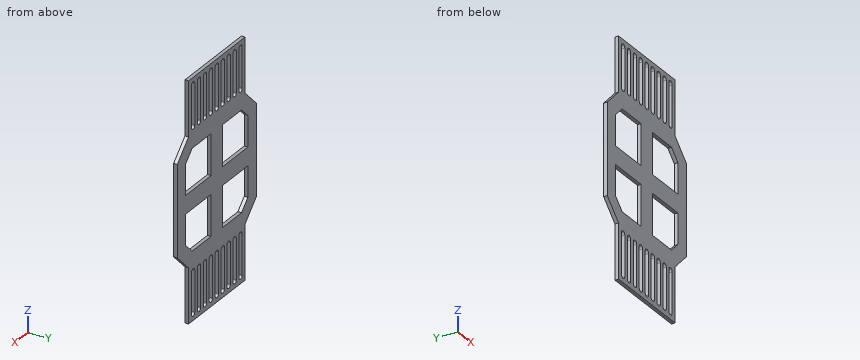
```python
from build123d import *

# Parameters (mm, degrees)
BOSS_EXTRUDE1_DEPTH = 2
CUT_EXTRUDE1_DEPTH  = 2
CIRPATTERN1_COUNT   = 4


with BuildPart() as part:
    # Sketch2 → Boss-Extrude1 (new body)
    with BuildSketch(Plane(origin=(0, 0, 0), x_dir=(1, 0, 0), z_dir=(0, 1, 0))):
        Polygon((-35, 35), (-25, 35), (-25, 65), (25, 65), (25, 35), (35, 35), (35, -35), (25, -35), (25, -65), (-25, -65), (-25, -35), (-35, -35), align=None)
        with BuildLine():
            Line((-1.5, 38.847241674), (-1.5, 61.152758326))
            ThreePointArc((-1.5, 61.152758326), (0, 62.652758326), (1.5, 61.152758326))
            Line((1.5, 61.152758326), (1.5, 38.847241674))
            ThreePointArc((1.5, 38.847241674), (0, 37.347241674), (-1.5, 38.847241674))
        make_face(mode=Mode.SUBTRACT)
        with BuildLine():
            Line((3.75, 38.847241674), (3.75, 61.152758326))
            ThreePointArc((3.75, 61.152758326), (5.25, 62.652758326), (6.75, 61.152758326))
            Line((6.75, 61.152758326), (6.75, 38.847241674))
            ThreePointArc((6.75, 38.847241674), (5.25, 37.347241674), (3.75, 38.847241674))
        make_face(mode=Mode.SUBTRACT)
        with BuildLine():
            Line((9, 38.847241674), (9, 61.152758326))
            ThreePointArc((9, 61.152758326), (10.5, 62.652758326), (12, 61.152758326))
            Line((12, 61.152758326), (12, 38.847241674))
            ThreePointArc((12, 38.847241674), (10.5, 37.347241674), (9, 38.847241674))
        make_face(mode=Mode.SUBTRACT)
        with BuildLine():
            Line((14.25, 38.847241674), (14.25, 61.152758326))
            ThreePointArc((14.25, 61.152758326), (15.75, 62.652758326), (17.25, 61.152758326))
            Line((17.25, 61.152758326), (17.25, 38.847241674))
            ThreePointArc((17.25, 38.847241674), (15.75, 37.347241674), (14.25, 38.847241674))
        make_face(mode=Mode.SUBTRACT)
        with BuildLine():
            Line((19.5, 38.847241674), (19.5, 61.152758326))
            ThreePointArc((19.5, 61.152758326), (21, 62.652758326), (22.5, 61.152758326))
            Line((22.5, 61.152758326), (22.5, 38.847241674))
            ThreePointArc((22.5, 38.847241674), (21, 37.347241674), (19.5, 38.847241674))
        make_face(mode=Mode.SUBTRACT)
        with BuildLine():
            Line((-6.75, 38.847241674), (-6.75, 61.152758326))
            ThreePointArc((-6.75, 61.152758326), (-5.25, 62.652758326), (-3.75, 61.152758326))
            Line((-3.75, 61.152758326), (-3.75, 38.847241674))
            ThreePointArc((-3.75, 38.847241674), (-5.25, 37.347241674), (-6.75, 38.847241674))
        make_face(mode=Mode.SUBTRACT)
        with BuildLine():
            Line((-12, 38.847241674), (-12, 61.152758326))
            ThreePointArc((-12, 61.152758326), (-10.5, 62.652758326), (-9, 61.152758326))
            Line((-9, 61.152758326), (-9, 38.847241674))
            ThreePointArc((-9, 38.847241674), (-10.5, 37.347241674), (-12, 38.847241674))
        make_face(mode=Mode.SUBTRACT)
        with BuildLine():
            Line((-17.25, 38.847241674), (-17.25, 61.152758326))
            ThreePointArc((-17.25, 61.152758326), (-15.75, 62.652758326), (-14.25, 61.152758326))
            Line((-14.25, 61.152758326), (-14.25, 38.847241674))
            ThreePointArc((-14.25, 38.847241674), (-15.75, 37.347241674), (-17.25, 38.847241674))
        make_face(mode=Mode.SUBTRACT)
        with BuildLine():
            Line((-22.5, 38.847241674), (-22.5, 61.152758326))
            ThreePointArc((-22.5, 61.152758326), (-21, 62.652758326), (-19.5, 61.152758326))
            Line((-19.5, 61.152758326), (-19.5, 38.847241674))
            ThreePointArc((-19.5, 38.847241674), (-21, 37.347241674), (-22.5, 38.847241674))
        make_face(mode=Mode.SUBTRACT)
        with BuildLine():
            Line((3.75, -38.847241674), (3.75, -61.152758326))
            ThreePointArc((3.75, -61.152758326), (5.25, -62.652758326), (6.75, -61.152758326))
            Line((6.75, -61.152758326), (6.75, -38.847241674))
            ThreePointArc((6.75, -38.847241674), (5.25, -37.347241674), (3.75, -38.847241674))
        make_face(mode=Mode.SUBTRACT)
        with BuildLine():
            Line((-1.5, -38.847241674), (-1.5, -61.152758326))
            ThreePointArc((-1.5, -61.152758326), (0, -62.652758326), (1.5, -61.152758326))
            Line((1.5, -61.152758326), (1.5, -38.847241674))
            ThreePointArc((1.5, -38.847241674), (0, -37.347241674), (-1.5, -38.847241674))
        make_face(mode=Mode.SUBTRACT)
        with BuildLine():
            Line((9, -38.847241674), (9, -61.152758326))
            ThreePointArc((9, -61.152758326), (10.5, -62.652758326), (12, -61.152758326))
            Line((12, -61.152758326), (12, -38.847241674))
            ThreePointArc((12, -38.847241674), (10.5, -37.347241674), (9, -38.847241674))
        make_face(mode=Mode.SUBTRACT)
        with BuildLine():
            Line((14.25, -38.847241674), (14.25, -61.152758326))
            ThreePointArc((14.25, -61.152758326), (15.75, -62.652758326), (17.25, -61.152758326))
            Line((17.25, -61.152758326), (17.25, -38.847241674))
            ThreePointArc((17.25, -38.847241674), (15.75, -37.347241674), (14.25, -38.847241674))
        make_face(mode=Mode.SUBTRACT)
        with BuildLine():
            Line((19.5, -38.847241674), (19.5, -61.152758326))
            ThreePointArc((19.5, -61.152758326), (21, -62.652758326), (22.5, -61.152758326))
            Line((22.5, -61.152758326), (22.5, -38.847241674))
            ThreePointArc((22.5, -38.847241674), (21, -37.347241674), (19.5, -38.847241674))
        make_face(mode=Mode.SUBTRACT)
        with BuildLine():
            Line((-6.75, -38.847241674), (-6.75, -61.152758326))
            ThreePointArc((-6.75, -61.152758326), (-5.25, -62.652758326), (-3.75, -61.152758326))
            Line((-3.75, -61.152758326), (-3.75, -38.847241674))
            ThreePointArc((-3.75, -38.847241674), (-5.25, -37.347241674), (-6.75, -38.847241674))
        make_face(mode=Mode.SUBTRACT)
        with BuildLine():
            Line((-12, -38.847241674), (-12, -61.152758326))
            ThreePointArc((-12, -61.152758326), (-10.5, -62.652758326), (-9, -61.152758326))
            Line((-9, -61.152758326), (-9, -38.847241674))
            ThreePointArc((-9, -38.847241674), (-10.5, -37.347241674), (-12, -38.847241674))
        make_face(mode=Mode.SUBTRACT)
        with BuildLine():
            Line((-17.25, -38.847241674), (-17.25, -61.152758326))
            ThreePointArc((-17.25, -61.152758326), (-15.75, -62.652758326), (-14.25, -61.152758326))
            Line((-14.25, -61.152758326), (-14.25, -38.847241674))
            ThreePointArc((-14.25, -38.847241674), (-15.75, -37.347241674), (-17.25, -38.847241674))
        make_face(mode=Mode.SUBTRACT)
        with BuildLine():
            Line((-22.5, -38.847241674), (-22.5, -61.152758326))
            ThreePointArc((-22.5, -61.152758326), (-21, -62.652758326), (-19.5, -61.152758326))
            Line((-19.5, -61.152758326), (-19.5, -38.847241674))
            ThreePointArc((-19.5, -38.847241674), (-21, -37.347241674), (-22.5, -38.847241674))
        make_face(mode=Mode.SUBTRACT)
    extrude(amount=BOSS_EXTRUDE1_DEPTH)

    # Sketch4 → Cut-Extrude1 (cut)
    with BuildSketch(Plane.XZ):
        Polygon((25, 35), (35, 25), (35, 35), align=None)
        Polygon((21.893398282, 27.5), (27.5, 21.893398282), (27.5, 5), (5, 5), (5, 27.5), align=None)
    cut_extrude1 = extrude(amount=-CUT_EXTRUDE1_DEPTH, mode=Mode.SUBTRACT)

    # CirPattern1: Cut-Extrude1 ×4 about axis
    cirpattern1_axis = Axis((0, 0, 0), (0, 1, 0))
    for i in range(1, CIRPATTERN1_COUNT):
        add(cut_extrude1.rotate(cirpattern1_axis, i * 360 / CIRPATTERN1_COUNT), mode=Mode.SUBTRACT)


solid = part.part
```
The model under review builds one solid part; all positions refer to its coordinate system, in mm. Round coordinates to 2 decimals unless told otherwise and drop trailing zeros. Order: outer loops, then holes, each group sorted by start corner. A loop starts at its lowest first (then second) coordinate and runs counter-clockwise, first axis right, second up.
(1) Wall thickness on L1, parallel to X at y = 1.1, z = 6; L2, parallel to Z at x = -13.5, y = 1.05; L3, parallel to X at y = 1.1, z = -24.5: over which ranges is each line inside the solid? List them lowest first.
Working result:
L1: x = -35 to -27.5, -5 to 5, 27.5 to 35
L2: z = -65 to -27.5, -5 to 5, 27.5 to 65
L3: x = -35 to -24.89, -5 to 5, 24.89 to 35
(2) For P1, Ø0.6, axis at y = 1, z = 48, coming from the +X side; P2, Ø0.6, axis at y = 1, z = 48, coming from the -X side, all flat-tipped, find the tip position at first contact; note any pin that passes through.
Working result:
P1: stops at x = 25
P2: stops at x = -25
(3) Take a section at D-D, the plane y = 1.45. Count the separate pieces of the cut face and the enclosed holes in it, plus the area to 3 significant figures.
Working result:
separate pieces: 1
enclosed holes: 22
area: 4,410 mm2
(4) Take a section at B-B, the plane x = 0. State the section outline as (y, z) points.
Working result:
outline: (0, -65) - (2, -65) - (2, -62.65) - (0, -62.65) - close; (0, -37.35) - (2, -37.35) - (2, 37.35) - (0, 37.35) - close; (0, 62.65) - (2, 62.65) - (2, 65) - (0, 65) - close
(5) Take a section at A-A, the plane z = 15.5. State the section outline as (x, y) points.
Working result:
outline: (-35, 0) - (-27.5, 0) - (-27.5, 2) - (-35, 2) - close; (-5, 0) - (5, 0) - (5, 2) - (-5, 2) - close; (27.5, 0) - (35, 0) - (35, 2) - (27.5, 2) - close
(6) Take a section at C-C, the plane x = 15.75. State the section outline as (y, z) points.
Working result:
outline: (0, -65) - (2, -65) - (2, -62.65) - (0, -62.65) - close; (0, -37.35) - (2, -37.35) - (2, -27.5) - (0, -27.5) - close; (0, -5) - (2, -5) - (2, 5) - (0, 5) - close; (0, 27.5) - (2, 27.5) - (2, 37.35) - (0, 37.35) - close; (0, 62.65) - (2, 62.65) - (2, 65) - (0, 65) - close
